Can you work these out from the drawing? Everything is in mm from the part's minimum corner. Round coordinates to 2 decimals unless told otherwise and drop trailing zeros. Loops run counter-clockwise (first coordinate to the right, second up) from the corner with the lowest first, then second, coordinate; pieces in that order, holes last. Notation, with made-up numbers: M 40,-14 L 62,-14 A7 cw 62,-10 Z; hole C -32,-24.75 d10. An arc over 180 degrees is marked long. Answer in a Markdown table with one row per item.
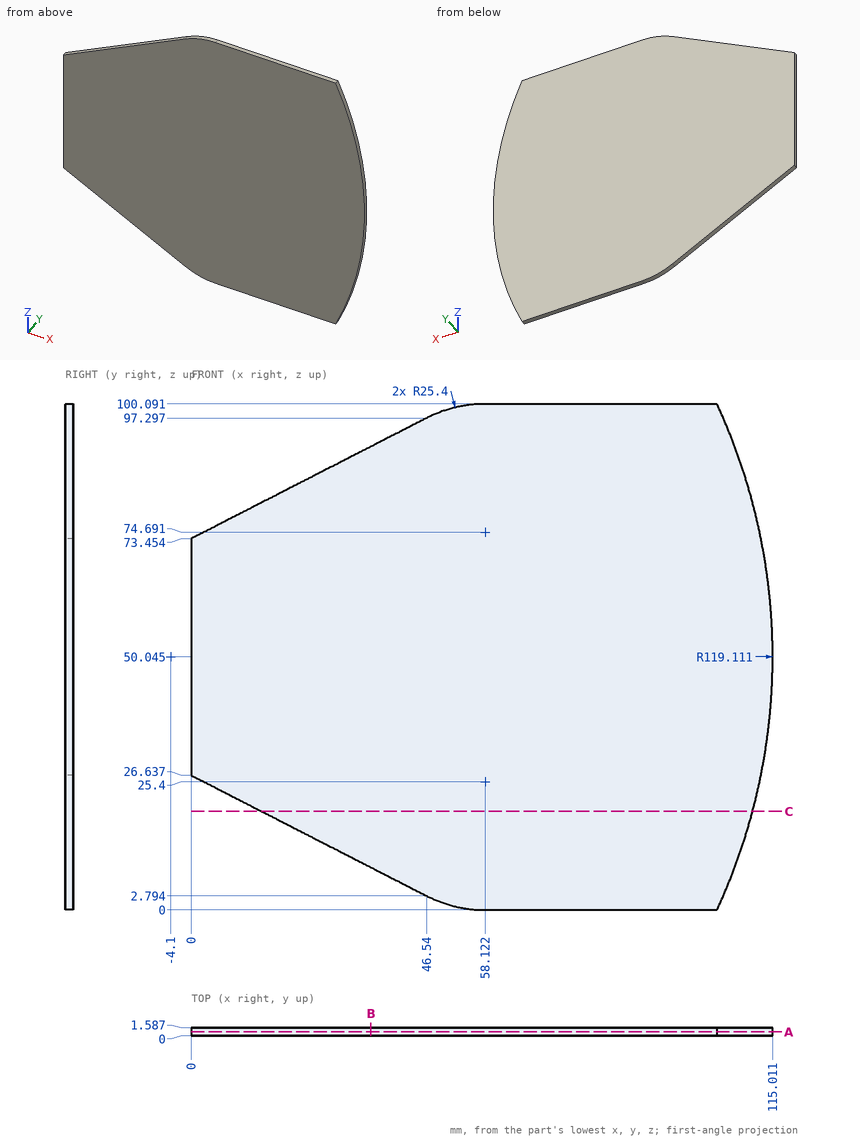
1) I want a section at A-A, the plane y = 0.8. Please give me the cut outline in (x, z) (1 decimal).
Computed:
| item | result |
|---|---|
| outline | M 0,26.6 L 46.5,2.8 A25.4 ccw 58.1,0 L 104,0 A119.1 ccw 104,100.1 L 58.1,100.1 A25.4 ccw 46.5,97.3 L 0,73.5 Z |
2) I need wall thicknesses on line 1 (X direction, y = 1.15, z = 40.5); line 2 (X direction, y = 0.1, z = 90) (1 decimal); line 3 (Z direction, x = 49, y = 1.05) (1 decimal). Which ranges of each line are inside material? Lowest first, please.
Computed:
| item | result |
|---|---|
| line 1 | x = 0 to 114.63 |
| line 2 | x = 32.3 to 108.1 |
| line 3 | z = 1.7 to 98.4 |
3) I want a section at C-C, the plane z = 19.5. Please give me the cut outline in (x, y), plus the area to 3 significant figures.
Computed:
| item | result |
|---|---|
| outline | M 13.93,0 L 111.03,0 L 111.03,1.59 L 13.93,1.59 Z |
| area | 154 mm² |
4) I want a section at B-B, the plane x = 35.5. Please give me the cut outline in (y, z).
Computed:
| item | result |
|---|---|
| outline | M 0,8.45 L 1.59,8.45 L 1.59,91.64 L 0,91.64 Z |
